```python
from build123d import *

# Parameters (mm, degrees)
CROQUIS1_R              = 12.5
SALIENTE_EXTRUIR1_DEPTH = 52
CROQUIS2_R              = 2.5
SALIENTE_EXTRUIR2_DEPTH = 3
CROQUIS3_R              = 1
SALIENTE_EXTRUIR3_DEPTH = 10
CROQUIS4_W              = 0.1
CROQUIS4_H              = 0.1
CORTAR_EXTRUIR1_DEPTH   = 0.1
CROQUIS5_W              = 1
CROQUIS5_H              = 0.1
CORTAR_EXTRUIR2_DEPTH   = 45


with BuildPart() as part:
    # Croquis1 → Saliente-Extruir1 (new body)
    with BuildSketch(Plane(origin=(0, 0, 0), x_dir=(1, 0, 0), z_dir=(0, 1, 0))):
        with Locations(Location((0, 0, 0), (0, 0, 90))):
            Circle(CROQUIS1_R)
    extrude(amount=SALIENTE_EXTRUIR1_DEPTH)

    # Croquis2 → Saliente-Extruir2 (add)
    with BuildSketch(Plane(origin=(0, 52, 0), x_dir=(1, 0, 0), z_dir=(0, 1, 0))):
        with Locations(Location((0, 0, 0), (0, 0, 270))):
            Circle(CROQUIS2_R)
    extrude(amount=SALIENTE_EXTRUIR2_DEPTH)

    # Croquis3 → Saliente-Extruir3 (add)
    with BuildSketch(Plane(origin=(0, 55, 0), x_dir=(1, 0, 0), z_dir=(0, 1, 0))):
        with Locations(Location((0, 0, 0), (0, 0, 270))):
            Circle(CROQUIS3_R)
    extrude(amount=SALIENTE_EXTRUIR3_DEPTH)

    # Croquis4 → Cortar-Extruir1 (cut)
    with BuildSketch(Plane(origin=(0, 52, 0), x_dir=(1, 0, 0), z_dir=(0, 1, 0))):
        with Locations((0, 12.5)):
            Rectangle(CROQUIS4_W, CROQUIS4_H)
    extrude(amount=-CORTAR_EXTRUIR1_DEPTH, mode=Mode.SUBTRACT)

    # Croquis5 → Cortar-Extruir2 (cut)
    with BuildSketch(Plane(origin=(0, 52, 0), x_dir=(1, 0, 0), z_dir=(0, 1, 0))):
        with Locations((0, 12.5)):
            Rectangle(CROQUIS5_W, CROQUIS5_H)
    extrude(amount=-CORTAR_EXTRUIR2_DEPTH, mode=Mode.SUBTRACT)


solid = part.part
```
Geometry check sheet. Reference: the model listing, model coordinates, mm. A direction names the side the tool comes from. Give positions to 0.01 mm unless a question says otherwise; leave off trailing zeros. Order: outer loops, then holes, each group sorted by start corner. A loop starts at its lowest first (then second) coordinate and runs counter-clockwise, first axis right, second up.
1. Access from +Z, -Z, +X, -X, +Y, -Y to the whole of each face (thin tool, end or side, straight path). Record for faces 1 (the face through (-3.755, 25.636, -11.923)), 2 (the face through (-2.44, 53.48, -0.54)).
2. Thickness scan on L1, parallel to Y at x = -10, z = 0.75; L2, parallel to Z at x = 7, y = 39; L3, parallel to Z at x = -4, y = 38. Record the ranges inside material, lowest first.
3. Section check C-C, the plane x = -7.5. Enter the section's corners in (y, z), and give its area (3 significant figures).
4. Gauge pin test, flat ends, axial feed: pin 1 Ø10 at (x, z) = (7.5, 1) entering from +Y; pin 2 Ø2 at (x, z) = (-6.5, 7.5) entering from -Y; pin 3 Ø4 at (x, z) = (-0.5, 3) entering from +Y; pin 4 Ø1.5 at (x, y) = (-4.5, 14) entering from +Z. Record the tip position at first contact, or that the pin passes through.
5. Section check A-A, the plane z = 0. Enter the section's corners in (x, y), and give its area (4 significant figures).
Values follow:
1. face 1: +Y, -Y
1. face 2: +Y
2. L1: y = 0 to 52
2. L2: z = -10.36 to 10.36
2. L3: z = -11.84 to 11.84
3. outline: (0, -10) - (52, -10) - (52, 10) - (0, 10) - close
3. area: 1,040 mm2
4. pin 1: stops at y = 52
4. pin 2: stops at y = 0
4. pin 3: stops at y = 55
4. pin 4: stops at z = 11.92
5. outline: (-12.5, 0) - (12.5, 0) - (12.5, 52) - (2.5, 52) - (2.5, 55) - (1, 55) - (1, 65) - (-1, 65) - (-1, 55) - (-2.5, 55) - (-2.5, 52) - (-12.5, 52) - close
5. area: 1,335 mm2
